Source: three-view drawing plus pictorial views. Frame: mm from the lowest corner of the part. Coordinates: 2 decimals unless noted, no trailing zeros. Order: outer loops, then holes, each group sorted by start corner. A loop starts at its lowest first (then second) coordinate and runs counter-clockwise, first axis right, second up. Notation, with made-up numbers: (72.5, -36.75) - (115.5, -36.75) arc R17 ccw to (115.5, -6.75) - close; hole circle Ø1 at (44.5, 25). An arc over 180 degrees is marked (long way). One line per question, with ' | ' between items.
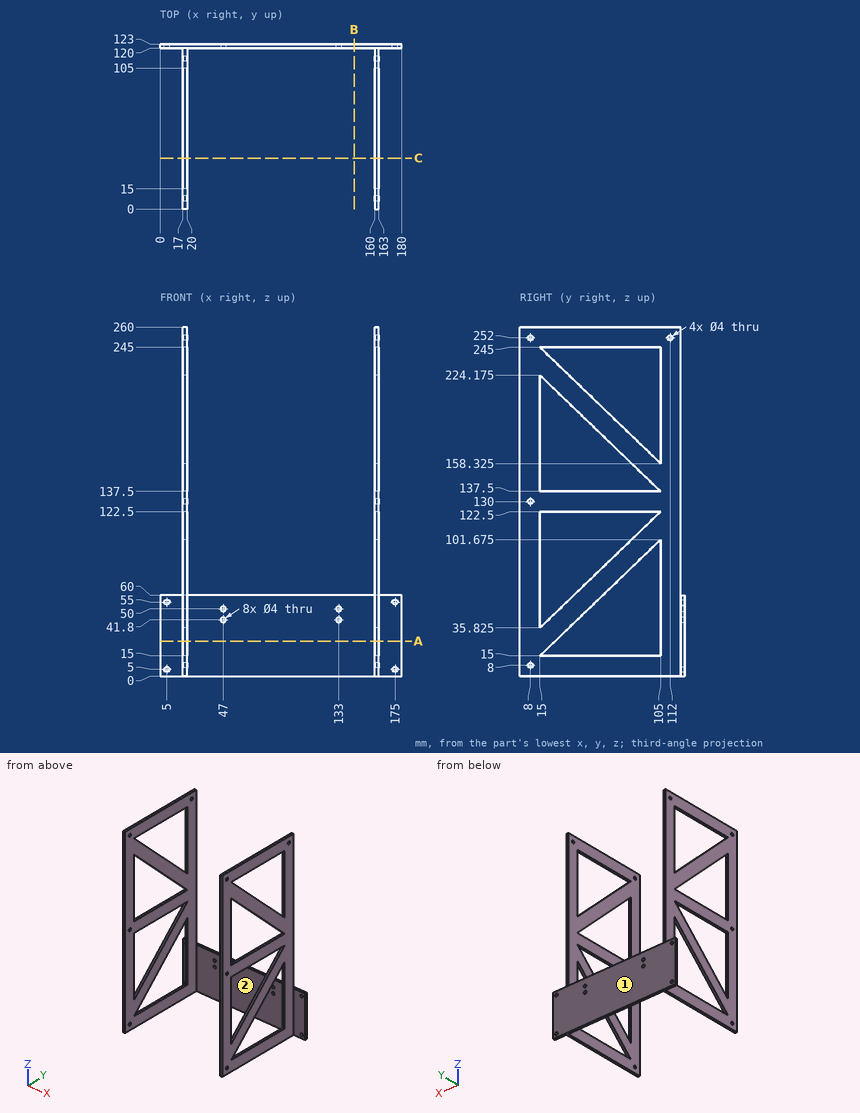
Item 1: Contact query for flat-ended pins moving along their axis: P1, Ø6.5, axis at y = 112, z = 252, coming from the +X side; P2, Ø3, axis at y = 82, z = 164, coming from the -X side; P3, Ø1.5, axis at x = 162, z = 183.5, coming from the +Y side. Output: stop coordinate, or through.
Data:
P1: x = 163 | P2: x = 17 | P3: y = 120
Item 2: Ray query, line 1 (Y direction, x = 161.4, z = 252); line 2 (Z direction, x = 175, y = 122.25); line 3 (X direction, y = 121, z = 55). Return the intervals inside material, ascending.
Data:
line 1: 0 to 6, 10 to 110, 114 to 120 | line 2: 0 to 3, 7 to 53, 57 to 60 | line 3: 0 to 3, 7 to 173, 177 to 180
Item 3: Section C-C on y = 38. Count the separate pieces of the cut face and the enclosed holes in it, and give its area (3 significant figures).
Data:
separate pieces: 10 | enclosed holes: 0 | area: 520 mm^2
Item 4: Draft query along X for the marked faces 1 and 2. Return one class per face: released by +X, released by -X, zero draft, split by the parting line, or undercut.
Data:
face 1: zero draft | face 2: undercut
Item 5: Section A-A on z = 26. Return the cut outline in (x, y), and give its area (3 significant figures).
Data:
outline: (0, 120) - (17, 120) - (17, 105) - (20, 105) - (20, 120) - (160, 120) - (160, 105) - (163, 105) - (163, 120) - (180, 120) - (180, 123) - (0, 123) - close; (17, 0) - (20, 0) - (20, 26.42) - (17, 26.42) - close; (160, 0) - (163, 0) - (163, 26.42) - (160, 26.42) - close | area: 789 mm^2
Item 6: Section B-B on x = 144.5. Return the cut outline in (y, z).
Data:
outline: (120, 0) - (123, 0) - (123, 60) - (120, 60) - close
